Design review of the part built by this model. Coordinates are the model's own, in mm. A direction names the side the tool comes from. Coordinates: 2 decimals unless noted, no trailing zeros. Order: outer loops, then holes, each group sorted by start corner. A loop starts at its lowest first (then second) coordinate and runs counter-clockwise, first axis right, second up. Notation, with made-up numbers: (62, 65) -> (90, 65) arc R12 ccw to (90, 76) -> close; hole circle Ø6 at (88, 54). An arc over 180 degrees is marked (long way). Write item = value, one per line.
```python
from build123d import *

# Parameters (mm, degrees)
BOSS_EXTRU_1_START      = -85
BOSS_EXTRU_1_DEPTH      = 280
ENL_V_MAT_EXTRU_1_DEPTH = 201.577291835
BOSS_EXTRU_2_REACH      = 203.42
CONG_1_R                = 5


with BuildPart() as part:
    # Esquisse1 → Boss.-Extru.1 (new body)
    with BuildSketch(Plane.XY.offset(BOSS_EXTRU_1_START)):
        Polygon((2, 1.5), (20, 1.5), (20, 0), (-20, 0), (-20, 1.5), (-2, 1.5), (-2, 41.5), (2, 41.5), align=None)
    extrude(amount=BOSS_EXTRU_1_DEPTH)

    # Esquisse3 → Enlèv. mat.-Extru.1 (cut, through all)
    with BuildSketch(Plane(origin=(2, 0, 0), x_dir=(0, 0, -1), z_dir=(1, 0, 0))):
        Polygon((-195, 41.5), (85, 41.5), (85, 30.743779015), (-195, 11.164271671), align=None)
    extrude(amount=-ENL_V_MAT_EXTRU_1_DEPTH, mode=Mode.SUBTRACT)

    # Boss.-Extru.2: up to this face of the body (flat: up to its plane)
    boss_extru_2_end = Plane(part.part.faces().sort_by_distance((-20, 0.75, 55))[0])
    # Esquisse2 → Boss.-Extru.2 (add, up to the picked face)
    with BuildSketch(Plane(origin=(20, 0, 0), x_dir=(0, 0, -1), z_dir=(1, 0, 0)), mode=Mode.PRIVATE) as boss_extru_2_sk1:
        with BuildLine():
            Line((-4.5, 0), (4.5, 0))
            Line((4.5, 0), (4.5, 20.289011459))
            ThreePointArc((4.5, 20.289011459), (0, 24.789011459), (-4.5, 20.289011459))
            Line((-4.5, 20.289011459), (-4.5, 0))
        make_face()
    boss_extru_2_tool1 = split(extrude(boss_extru_2_sk1.sketch, amount=-BOSS_EXTRU_2_REACH, mode=Mode.PRIVATE), bisect_by=boss_extru_2_end, keep=Keep.BOTH, mode=Mode.PRIVATE)
    add(boss_extru_2_tool1.solids().sort_by(Axis((20, 11.932824, 0), (-1, 0, 0)))[0])

    # Congé1
    cong_1_edges = [part.edges().sort_by_distance(p)[0] for p in [
        (-20, 0.75, 195),
        (20, 0.75, 195),
        (0, 30.743779015, -85),
        (0, 11.164271671, 195),
        (20, 0.75, -85),
        (-20, 0.75, -85),
    ]]
    fillet(cong_1_edges, radius=CONG_1_R)


solid = part.part
```
(1) For L1, parallel to X at y = 16, z = -40; L2, parallel to Z at x = 15, y = 16.5; L3, parallel to Y at x = -5, z = 65.5, list the stretches that pass through material, from the lowest coordinate up.
Report:
L1 = -2 to 2
L2 = -4.5 to 4.5
L3 = 0 to 1.5
(2) For faces 1 (the flat face through (-11, 11, -4.5)), 2 (the cylindrical face through (11.126, 24.788, -0.099)), 3 (the flat face through (-11, 11, 4.5)), list the 3-axis set-ups (+Z, -Z, +X, -X, +Y, -Y) from which the entire face can be reached by the end or side of a thin tool; tool diameter is ignored.
Report:
face_1 = -Z, -X, +Y
face_2 = +X, +Y
face_3 = +Z, -X, +Y
(3) We need section A-A (x = 10). Write out the cut boundary in (y, z), and give its area (3 significant figures).
Report:
outline = (0, -85) -> (1.5, -85) -> (1.5, -4.5) -> (20.29, -4.5) arc R4.5 ccw to (20.29, 4.5) -> (1.5, 4.5) -> (1.5, 195) -> (0, 195) -> close
area = 621 mm²
(4) We need section C-C (y = 18). Write out the cut boundary in (x, z), and give its area (3 significant figures).
Report:
outline = (-20, -4.5) -> (-2, -4.5) -> (-2, -85) -> (2, -85) -> (2, -4.5) -> (20, -4.5) -> (20, 4.5) -> (2, 4.5) -> (2, 97.24) -> (-2, 97.24) -> (-2, 4.5) -> (-20, 4.5) -> close
area = 1,050 mm²
(5) We need section B-B (z = 124.5). Write out the cut boundary in (x, y).
Report:
outline = (-20, 0) -> (20, 0) -> (20, 1.5) -> (2, 1.5) -> (2, 16.09) -> (-2, 16.09) -> (-2, 1.5) -> (-20, 1.5) -> close
(6) Insertion check: pin 1 (5.5 mm diameter, centred on x = -9, z = 127, fed in from +Y); pin 2 (6 mm diameter, centred on x = 4, z = 114.5, fed in from +Y); pin 3 (2 mm diameter, centred on y = 4.5, z = 45.5, fed in from +X). Each pin has a flat end and moves straight along its axis. Give the tip position at first contact, or say it passes through.
Report:
pin_1 = 1.5
pin_2 = 16.95
pin_3 = 2
